```python
from build123d import *

# Parameters (mm, degrees)
BOSS_EXTRUDE1_DEPTH = 2
BOSS_EXTRUDE2_DEPTH = 3
SKETCH3_W           = 7
SKETCH3_H           = 3.108863517
BOSS_EXTRUDE3_DEPTH = 2


with BuildPart() as part:
    # Sketch1 → Boss-Extrude1 (new body)
    with BuildSketch(Plane(origin=(0, 0, 0), x_dir=(1, 0, 0), z_dir=(0, 1, 0))):
        Polygon((-7.5, -4.5), (7.5, -4.5), (11.4, -4.5), (11.4, 4.5), (7.5, 4.5), (-7.5, 4.5), (-7.5, 5.5), (-14.5, 5.5), (-14.5, -5.5), (-7.5, -5.5), align=None)
    extrude(amount=BOSS_EXTRUDE1_DEPTH)

    # Sketch2 → Boss-Extrude2 (add)
    with BuildSketch(Plane(origin=(0, 0, 0), x_dir=(1, 0, 0), z_dir=(0, 1, 0))):
        Polygon((6.1, 4.5), (-7.5, 4.5), (-7.5, 5.5), (-14.5, 5.5), (-14.5, 3.5), (0.5, 3.5), (0.5, 3), (6.1, 3), align=None)
        Polygon((-7.5, -4.5), (-7.5, -5.5), (-14.5, -5.5), (-14.5, -3.5), (0.5, -3.5), (0.5, -3), (7.5, -3), (9.9, -3), (9.9, 4.5), (11.4, 4.5), (11.4, -4.5), (7.5, -4.5), align=None)
        Polygon((0.5, -1.6), (0.5, 1.6), (7.5, 1.6), (7.5, 4.5), (8.5, 4.5), (8.5, -1.6), (7.5, -1.6), align=None)
    extrude(amount=-BOSS_EXTRUDE2_DEPTH)

    # Sketch3 → Boss-Extrude3 (add)
    with BuildSketch(Plane.XZ.offset(3)):
        with Locations((-11, 3.945568242)):
            Rectangle(SKETCH3_W, SKETCH3_H)
        with Locations((-11, -3.945568242)):
            Rectangle(SKETCH3_W, SKETCH3_H)
    extrude(amount=-BOSS_EXTRUDE3_DEPTH)


solid = part.part
```
The listing builds one solid part. Answer for the finished solid, in the listing's coordinates (mm). A direction names the side the tool comes from. Coordinates: 2 decimals unless noted, no trailing zeros. Write each loop counter-clockwise with the first axis right and the second up, starting at its lowest first coordinate (ties: lowest second). Pieces come first, ordered by that corner, then holes. Notation, with made-up numbers: (16.25, 10.5) - (64.25, 10.5) arc R22 ccw to (64.25, 30.5) - close; hole circle Ø9 at (43, 44). An arc over 180 degrees is marked (long way). Return JSON: item names as keys, results as strings. Group by question number.
Q1. Flat-ended cylindrical pins translate along their axes: pin 1 Ø2.5 at (x, y) = (5, -1) entering from -Z; pin 2 Ø2.5 at (x, y) = (5, 0) entering from +Z; pin 3 Ø0.5 at (y, z) = (-1, -5) entering from +X. Find the tip coordinate at first contact, or state that the pin passes through.
Q2. Find the intervals of material crossed by line 1 along Z through (x, y) = (2, -1.9); line 2 along Z through (x, y) = (-11.25, -1.85); line 3 along X through (y, z) = (-2.45, 2.5), in increasing order. Write a range as [from, to].
Q3. The part is cut by section C-C on x = -10. Write down the section's boundary in (y, z).
Q4. The part is cut by section A-A on y = -1.95. Write down the section's boundary in (x, z).
Q5. The part is cut by section B-B on z = -4.25. Write down the section's boundary in (x, y).
Q6. The part is cut by section D-D on y = 0.9. Write down the section's boundary in (x, z), and give its area (3 significant figures).
Q7. For a pull along Y with two mould halves and no side action, classify faces 6 (the flat face through (-5, -1, 3.5)), 7 (the flat face through (0, -3, 4)), 8 (the flat face through (11.4, -1, 0)) as +Y half, -Y half, draft (parallel to the pull), parting line (faces both ways), or undercut.
Q8. Which of the six approach directions +Z, -Z, +X, -X, +Y, -Y give full straight-line access (tool end or side, diameter ignored) to faces 1 (the flat face through (-11, -2, 2.391)), 2 (the flat face through (-5, -1, -3.5)), 3 (the flat face through (-11, -1, -3)), 4 (the flat face through (6.1, -1, -4)), 5 (the flat face through (5, -1, 3))?
Evaluation:
{
 "1": {"pin 1": "stops at z = -4.5", "pin 2": "stops at z = 4.5", "pin 3": "stops at x = -7.5"},
 "2": {"line 1": "z = [-4.5, -3], [-1.6, 1.6], [3, 4.5]", "line 2": "z = [-5.5, -2.39], [2.39, 5.5]", "line 3": "x = [-14.5, -7.5], [9.9, 11.4]"},
 "3": {"outline": "(-3, -5.5) - (2, -5.5) - (2, 5.5) - (-3, 5.5) - (-3, 2.39) - (-1, 2.39) - (-1, 3.5) - (0, 3.5) - (0, -3.5) - (-1, -3.5) - (-1, -2.39) - (-3, -2.39) - close"},
 "4": {"outline": "(-14.5, -5.5) - (-7.5, -5.5) - (-7.5, -4.5) - (6.1, -4.5) - (6.1, -3) - (0.5, -3) - (0.5, -3.5) - (-7.5, -3.5) - (-7.5, -2.39) - (-14.5, -2.39) - close; (-14.5, 2.39) - (-7.5, 2.39) - (-7.5, 3.5) - (0.5, 3.5) - (0.5, 3) - (9.9, 3) - (9.9, -4.5) - (11.4, -4.5) - (11.4, 4.5) - (-7.5, 4.5) - (-7.5, 5.5) - (-14.5, 5.5) - close; (0.5, -1.6) - (7.5, -1.6) - (7.5, -4.5) - (8.5, -4.5) - (8.5, 1.6) - (0.5, 1.6) - close"},
 "5": {"outline": "(-14.5, -3) - (6.1, -3) - (6.1, 0) - (7.5, 0) - (7.5, -3) - (8.5, -3) - (8.5, 0) - (9.9, 0) - (9.9, -3) - (11.4, -3) - (11.4, 2) - (-14.5, 2) - close"},
 "6": {"outline": "(-14.5, -5.5) - (-7.5, -5.5) - (-7.5, -4.5) - (11.4, -4.5) - (11.4, 4.5) - (-7.5, 4.5) - (-7.5, 5.5) - (-14.5, 5.5) - close", "area": "247 mm2"},
 "7": {"face 6": "undercut", "face 7": "-Y half", "face 8": "draft"},
 "8": {"face 1": "-X, -Y", "face 2": "none", "face 3": "-X", "face 4": "-Z, -Y", "face 5": "-Y"}
}
